Check sheet for the modelled part. Datum: model origin and axes. Units: mm. A direction names the side the tool comes from. Round coordinates to 2 decimals unless told otherwise and drop trailing zeros. Order: outer loops, then holes, each group sorted by start corner. A loop starts at its lowest first (then second) coordinate and runs counter-clockwise, first axis right, second up.
from build123d import *

# Parameters (mm, degrees)
SKETCH1_R           = 3
BOSS_EXTRUDE1_DEPTH = 6
CHAMFER1_SIZE       = 6
SKETCH2_R           = 8.1
CUT_EXTRUDE1_DEPTH  = 5


with BuildPart() as part:
    # Sketch1 → Boss-Extrude1 (new body)
    with BuildSketch(Plane(origin=(0, 0, 0), x_dir=(1, 0, 0), z_dir=(0, 1, 0))):
        Polygon((0, 0), (32, 0), (32, 20), (26, 20), (26, 42), (0, 42), align=None)
        with Locations(Location((22, 10, 0), (0, 0, 270))):
            Circle(SKETCH1_R, mode=Mode.SUBTRACT)
    extrude(amount=BOSS_EXTRUDE1_DEPTH)

    # Chamfer1
    chamfer1_edges = [part.edges().sort_by_distance(p)[0] for p in [
        (32, 3, -20),
        (32, 3, 0),
    ]]
    chamfer(chamfer1_edges, length=CHAMFER1_SIZE - 0.0001)  # a hair under: the kernel refuses the full size

    # Sketch2 → Cut-Extrude1 (cut)
    with BuildSketch(Plane(origin=(0, 6, 0), x_dir=(1, 0, 0), z_dir=(0, 1, 0))):
        with Locations(Location((22, 10, 0), (0, 0, 270))):
            Circle(SKETCH2_R)
    extrude(amount=-CUT_EXTRUDE1_DEPTH, mode=Mode.SUBTRACT)


solid = part.part
1) Gauge pin test, flat ends, axial feed: pin 1 (2 mm diameter, centred on y = 3, z = -17.5, fed in from +X); pin 2 (13 mm diameter, centred on x = 22, z = -11, fed in from +Y); pin 3 (3.5 mm diameter, centred on x = 22, z = -10, fed in from +Y); pin 4 (3 mm diameter, centred on y = 3, z = -25.5, fed in from +X). Record the tip position at first contact, or that the pin passes through.
2) Sectioned sample at D-D on z = -22. Record the cut outline in (x, y), and give its area (3 significant figures).
3) Set-up check for faces 4 (the face through (22.1, 1, -6.5)), 5 (the face through (26, 3, -31)), 6 (the face through (13, 3, -42)): record each of +Z, -Z, +X, -X, +Y, -Y from which the full face is reachable in a straight line by a thin tool's end or side.
4) Scan lines: line 1 (X direction, y = 3.95, z = -10); line 2 (X direction, y = 0.65, z = -10); line 3 (Z direction, x = 22, y = 0.3). Record each from-to range of solid material in increasing order.
5) Sectioned sample at B-B on z = -10. Record the cut outline in (x, y), and give its area (3 significant figures).
6) Draft check along X on faces 1 (the face through (22.1, 0.5, -13)), 2 (the face through (29, 3, -17)), 3 (the face through (12, 6, -21)). Enter one of: pulls with the +X half, pulls with the -X half, needs draft (parallel to the pull), parting line crosses it, or undercut.
7) Sectioned sample at A-A on x = 22. Record the cut outline in (y, z).
Values found:
1. pin 1: stops at x = 29.5
1. pin 2: stops at y = 1
1. pin 3: passes through
1. pin 4: stops at x = 26
2. outline: (0, 0) - (26, 0) - (26, 6) - (0, 6) - close
2. area: 156 mm2
3. face 4: +Y
3. face 5: -Z, +X, +Y, -Y
3. face 6: -Z, +X, -X, +Y, -Y
4. line 1: x = 0 to 13.9, 30.1 to 32
4. line 2: x = 0 to 19, 25 to 32
4. line 3: z = -42 to -13, -7 to 0
5. outline: (0, 0) - (19, 0) - (19, 1) - (13.9, 1) - (13.9, 6) - (0, 6) - close; (25, 0) - (32, 0) - (32, 6) - (30.1, 6) - (30.1, 1) - (25, 1) - close
5. area: 105 mm2
6. face 1: undercut
6. face 2: pulls with the +X half
6. face 3: needs draft
7. outline: (0, -42) - (6, -42) - (6, -18.1) - (1, -18.1) - (1, -13) - (0, -13) - close; (0, -7) - (1, -7) - (1, -1.9) - (6, -1.9) - (6, 0) - (0, 0) - close
